Source: CAD feature listing. Evaluate the final solid. Frame: model axes, mm. Give positions to 0.01 mm unless a question says otherwise; leave off trailing zeros. Write each loop counter-clockwise with the first axis right and the second up, starting at its lowest first coordinate (ties: lowest second). Pieces come first, ordered by that corner, then holes.
```python
from build123d import *

# Parameters (mm, degrees)
EXTRUDE_1_DEPTH = 5


with BuildPart() as part:
    # Эскиз1 → Бобышка-Вытянуть1 (new body)
    with BuildSketch(Plane.XY):
        with BuildLine():
            ThreePointArc((-3, 12.562492976), (-4.5, 11.062492976), (-3, 9.562492976))
            Line((-3, 9.562492976), (-2.5, 9.562492976))
            Line((-2.5, 9.562492976), (-2.5, 4.062492976))
            Line((-2.5, 4.062492976), (-6, 4.062492976))
            Line((-6, 4.062492976), (-62.5, 4.062492976))
            Line((-62.5, 4.062492976), (-62.5, 15.062492976))
            ThreePointArc((-62.5, 15.062492976), (-32.684005961, 20.119684505), (-2.5, 21.989034877))
            Line((-2.5, 21.989034877), (-2.5, 12.562492976))
            Line((-2.5, 12.562492976), (-3, 12.562492976))
        make_face()
    extrude(amount=EXTRUDE_1_DEPTH)


solid = part.part
```
1. Cut plane C-C, the plane y = 10.25. Return the cut outline in (x, z), then the cut area to 3 significant figures.
2. Contact query for a flat-ended pin moving along its axis: P1, Ø2, axis at x = -9.5, z = 1, coming from the +Y side. Output: stop coordinate, or through.
3. Mould query, pull axis Y, two halves, no side actions, for faces 1 (the flat face through (-32, 4.062, 2)), 2 (the flat face through (-32, 13, 0)), 3 (the cylindrical face through (-4.5, 11.1, 2.5)). Classes: +Y half, -Y half, draft (parallel to the pull), parting line (faces both ways), or undercut.
4. Line query: L1, parallel to X at y = 11, z = 0.7; L2, parallel to Y at x = -46.5, z = 2.2; L3, parallel to Y at x = -21, z = 1.3. Output: solid intervals per line, ascending.
5. Cut plane B-B, the plane x = -14.5. Return the cut outline in (y, z), then the cut area to 3 significant figures.
6. Cut plane A-A, the plane z = 2.5. Return the cut outline in (x, y).
Response values:
1. outline: (-62.5, 0) - (-4.26, 0) - (-4.26, 5) - (-62.5, 5) - close
1. area: 291 mm2
2. P1: stops at y = 21.87
3. face 1: -Y half
3. face 2: draft
3. face 3: undercut
4. L1: x = -62.5 to -4.5
4. L2: y = 4.06 to 18.18
4. L3: y = 4.06 to 21.23
5. outline: (4.06, 0) - (21.63, 0) - (21.63, 5) - (4.06, 5) - close
5. area: 87.8 mm2
6. outline: (-62.5, 4.06) - (-2.5, 4.06) - (-2.5, 9.56) - (-3, 9.56) arc R1.5 cw to (-3, 12.56) - (-2.5, 12.56) - (-2.5, 21.99) arc R285 ccw to (-62.5, 15.06) - close
